Verification items for the finished model (mm, model axes). Give positions to 0.01 mm unless a question says otherwise; leave off trailing zeros. Loops run counter-clockwise (first coordinate to the right, second up) from the corner with the lowest first, then second, coordinate; pieces in that order, holes last. Notation, with made-up numbers: (-19.5, 89) - (35.5, 89) arc R36 cw to (35.5, 123) - close; hole circle Ø7 at (-3, 83.25). An arc over 180 degrees is marked (long way). One line per question, with ' | ' between items. Start each with the question number.
1. Section check C-C, the plane z = -0.25. Enter the section's corners in (x, y), then the cut area to 3 significant figures.
2. Depth check by flat-ended pin: pin 1 Ø8 at (x, z) = (-56.5, 13) entering from +Y; pin 2 Ø4 at (x, z) = (-50.5, -2.5) entering from -Y; pin 3 Ø1.5 at (x, y) = (-55.5, 26) entering from +Z. Enter the tip coordinate at first touch or a pass-through.
3. Section check A-A, the plane y = 20.7. Enter the section's corners in (x, z), then the cut area to 3 significant figures.
4. Mould release check, pull along Z, two halves, no side actions. Record for faces 1 (the face through (-55, 21, -5)), 2 (the face through (-52.9, 20.8, 5)), 3 (the face through (-57.11, 20.79, 9.93)): +Z half, -Z half, draft (parallel to the pull), parting line (faces both ways), or undercut.
5. Section check B-B, the plane z = 8.5. Enter the section's corners in (x, y).
6. Thickness scan on line 1 along Z through (x, y) = (-52.75, 26.25); line 2 along Y through (x, z) = (-54.75, -1.5); line 3 along Z through (x, y) = (-45.5, 14.75). Record the ranges inside material, lowest first. Write a range as from..to.
from build123d import *

# Parameters (mm, degrees)
SKETCH1_R           = 12.5
BOSS_EXTRUDE1_DEPTH = 5
CHAMFER1_SIZE       = 2
SKETCH2_R           = 2
BOSS_EXTRUDE2_DEPTH = 10


with BuildPart() as part:
    # Sketch1 → Boss-Extrude1 (new, symmetric)
    with BuildSketch(Plane.XY):
        with Locations((-55.110705908, 20.7)):
            Circle(SKETCH1_R)
    extrude(amount=BOSS_EXTRUDE1_DEPTH, both=True)

    # Chamfer1
    chamfer1_edges = [part.edges().sort_by_distance(p)[0] for p in [
        (-67.610705908, 20.7, -5),
        (-67.610705908, 20.7, 5),
    ]]
    chamfer(chamfer1_edges, length=CHAMFER1_SIZE)

    # Sketch2 → Boss-Extrude2 (add)
    with BuildSketch(Plane.XY.offset(5)):
        with Locations((-55.110705908, 20.7)):
            Circle(SKETCH2_R)
    extrude(amount=BOSS_EXTRUDE2_DEPTH)


solid = part.part
Results list:
1) outline: circle Ø25 at (-55.11, 20.7) | area: 491 mm²
2) pin 1: y = 22.7 | pin 2: y = 8.48 | pin 3: z = 5
3) outline: (-67.61, -3) - (-65.61, -5) - (-44.61, -5) - (-42.61, -3) - (-42.61, 3) - (-44.61, 5) - (-53.11, 5) - (-53.11, 15) - (-57.11, 15) - (-57.11, 5) - (-65.61, 5) - (-67.61, 3) - close | area: 282 mm²
4) face 1: -Z half | face 2: +Z half | face 3: draft
5) outline: circle Ø4 at (-55.11, 20.7)
6) line 1: -5..5 | line 2: 8.21..33.19 | line 3: -4.2..4.2
